Part model, mm, in its own coordinate system. A direction names the side the tool comes from. Coordinates: 2 decimals unless noted, no trailing zeros. Loops run counter-clockwise (first coordinate to the right, second up) from the corner with the lowest first, then second, coordinate; pieces in that order, holes last. Notation, with made-up numbers: M 72.5,19.25 L 128.5,19.25 A33 cw 128.5,57.25 Z; hole C 63.5,-14 d3. An arc over 180 degrees is marked long. Answer as a JSON object with one key per item and string values. Group by question number.
1. Drop flat-ended pins along their axis: pin 1 Ø0.6 at (y, z) = (4, -2.5) entering from -X; pin 2 Ø2 at (x, z) = (3, -2) entering from -Y; pin 3 Ø1.6 at (x, y) = (17, 5.5) entering from -Z. Give the stop position or say it passes through.
2. Mould opens along Y. For faces 6 (the face through (16.6, 2.7, -2.2)), 7 (the face through (17, 7, -2.2)) say: released by +Y, released by -Y, zero draft, split by the parting line, or undercut.
3. 3-axis set-ups, long thin cutter, end or side, ignore diameter. For faces 1 (the face through (1.6, 0.3, 3.05)), 2 (the face through (16.5, 5.3, -2.2)), 3 (the face through (16.5, 5.3, 2.2)), 4 (the face through (17, 7, 2.2)), 5 (the face through (1, 0, 2.75)): which of +Z, -Z, +X, -X, +Y, -Y reach the whole face in a straight line?
4. Drill centre lines: L1, parallel to Z at x = 17.5, y = 2.5; L2, parallel to Y at x = 16.55, z = 2.4; L3, parallel to Y at x = 1.65, z = 2.95. Where is each one in solid material? Low to high.
5. Saw through at D-D on x = 13.75. Write the cut outline in (y, z), then the cut area to 3 significant figures.
6. Saw through at C-C on y = 5.25. Write the cut outline in (x, z), then the cut area to 3 significant figures.
7. Saw through at B-B on y = -0.75. Write the cut outline in (x, z).
8. Saw through at A-A on z = 0.75. Write the cut outline in (x, y).
Autodesk Inventor part; units mm, degrees
ref_plane "YZ Plane" through (0, 0, 0) normal (1, 0, 0) x (0, 1, 0)
ref_plane "XZ Plane" through (0, 0, 0) normal (0, 1, 0) x (-1, 0, 0)
ref_plane "XY Plane" through (0, 0, 0) normal (0, 0, 1) x (1, 0, 0)
sketch "Sketch1" plane through (0, 0, 0) normal (1, 0, 0) x (0, 1, 0)
  line L0 (1.75, 3.05) -> (-2.05, 3.05)
  line L1 (-2.05, 3.05) -> (-2.05, 2.75)
  line L2 (-2.05, 2.75) -> (1.45, 2.75)
  line L3 (1.45, 2.75) -> (1.45, -2.75)
  line L4 (1.45, -2.75) -> (-2.05, -2.75)
  line L5 (-2.05, -2.75) -> (-2.05, -3.05)
  line L6 (-2.05, -3.05) -> (1.75, -3.05)
  line L7 (1.75, -3.05) -> (1.75, 3.05)
  point P0 (0, 0)
  dimension "d0" = 0.3
  dimension "d1" = 0.3
  dimension "d2" = 0.3
  dimension "d4" = 3.5
  dimension "d15" = 6.1
  dimension "d16" = 3.05
  dimension "d17" = 1.75
extrude "Extrusion1" add sketch "Sketch1" along normal blind 3.3
fillet "Fillet1" radius 1.6 4 edges at (3.3, -2.05, 2.9) (0, -2.05, 2.9) (0, -2.05, -2.9) (3.3, -2.05, -2.9)
sketch "Sketch2" plane through (0, 1.75, 3.05) normal (0, 0, 1) x (1, 0, 0)
  arc A0 (1.7, -3.8) -> (3.3, -2.2) centre (1.7, -2.2) ccw
  arc A1 (0, -2.2) -> (1.6, -3.8) centre (1.6, -2.2) ccw
  line L0 (1.6, -2.2) -> (1.7, -2.2)
  point P0 (0, -1.75)
  point P1 (1.65, -2.2)
hole "Hole1" at (1.65, -0.45, 3.05) direction (0, 0, -1) diameter 1 end through all
sketch "Sketch3" plane through (3.3, 0, 0) normal (1, 0, 0) x (0, 0, -1)
  line L0 (3.05, 1.75) -> (-3.05, 1.75)
  line L1 (0, 1.75) -> (0, 1.45)
  line L2 (-2.75, 1.45) -> (2.75, 1.45)
  line L3 (2, 1.45) -> (-2, 1.45)
  line L4 (-2, 1.45) -> (-2, 1.75)
  line L5 (-2, 1.75) -> (2, 1.75)
  line L6 (2, 1.75) -> (2, 1.45)
  line L7 (2, 1.45) -> (-2, 1.75) construction
  line L8 (-2, 1.45) -> (2, 1.75) construction
  point P0 (0, 0)
  point P1 (0, 1.6)
  dimension "d18" = 4
extrude "Extrusion2" add sketch "Sketch3" along normal blind 15.25
sketch "Sketch4" plane through (18.55, 0, 0) normal (1, 0, 0) x (0, 0, -1)
  line L0 (-2.75, 1.45) -> (2.75, 1.45)
  line L1 (0, 1.45) -> (0, 1.75)
  line L2 (3.05, 1.75) -> (-3.05, 1.75)
  line L3 (2.5, 1.45) -> (-2.5, 1.45)
  line L4 (-2.5, 1.45) -> (-2.5, 1.75)
  line L5 (-2.5, 1.75) -> (2.5, 1.75)
  line L6 (2.5, 1.75) -> (2.5, 1.45)
  line L7 (2.5, 1.45) -> (-2.5, 1.75) construction
  line L8 (-2.5, 1.45) -> (2.5, 1.75) construction
  line L9 (-2.5, 1.75) -> (-2.2, 1.75)
  line L10 (-2.2, 1.75) -> (-2.2, 6.75)
  line L11 (-2.2, 6.75) -> (-2.5, 6.75)
  line L12 (-2.5, 6.75) -> (-2.5, 1.75)
  line L13 (2.5, 1.75) -> (2.2, 1.75)
  line L14 (2.2, 1.75) -> (2.2, 6.75)
  line L15 (2.2, 6.75) -> (2.5, 6.75)
  line L16 (2.5, 6.75) -> (2.5, 1.75)
  point P0 (0, 0)
  point P1 (0, 1.6)
  dimension "d21" = 5
  dimension "d22" = 0.3
  dimension "d23" = 0.3
  dimension "d24" = 5
extrude "Extrusion3" add sketch "Sketch4" against normal blind 4
fillet "Fillet2" radius 2 4 edges at (18.55, 6.75, 2.35) (14.55, 6.75, 2.35) (14.55, 6.75, -2.35) (18.55, 6.75, -2.35)
sketch "Sketch5" plane through (14.55, 1.45, 2.5) normal (0, 0, 1) x (1, 0, 0)
  arc A0 (4, 3.3) -> (0, 3.3) centre (2, 3.3) ccw
  point P0 (-14.55, -1.45)
  point P1 (2, 3.8)
  dimension "d35" = 0.5
hole "Hole2" at (16.55, 5.25, 2.5) direction (0, 0, -1) diameter 1 end through all
sketch "Sketch6" plane through (14.55, 1.75, -2.2) normal (0, 0, 1) x (1, 0, 0)
  circle A0 centre (2, 3.5) radius 0.5
  circle A1 centre (2, 3.5) radius 0.5
  circle A2 centre (2, 3.5) radius 2.25
  point P0 (-14.55, -1.75)
  dimension "d36" = 4.5
extrude "Extrusion4" add sketch "Sketch6" along normal blind 4.4 contours A0 | A2
ref_plane "Work Plane1" through (-1.2438, 1.2458, -3.05) normal (-0.9978, 0.0664, 0) x (-0.0664, -0.9978, 0)
sketch "Sketch7" plane through (-1.2438, 1.2458, -3.05) normal (-0.9978, 0.0664, 0) x (-0.0664, -0.9978, 0)
  circle A0 centre (-6.8395, 3.05) radius 0.875
  point P0 (1.1605, 3.05)
  dimension "d39" = 1.75
  dimension "d40" = 8
properties part number "Arm"
Outcome:
{
 "1": {"pin 1": "stops at x = 14.55", "pin 2": "stops at y = -1.92", "pin 3": "stops at z = -2.5"},
 "2": {"face 6": "undercut", "face 7": "zero draft"},
 "3": {"face 1": "+Z, +X, -X, +Y, -Y", "face 2": "-Z", "face 3": "+Z", "face 4": "+Z, +Y", "face 5": "+X, -X, -Y"},
 "4": {"L1": "z = -2.5 to -2.2, 2.2 to 2.5", "L2": "y = 1.45 to 4.75, 5.75 to 6.75", "L3": "y = -2.05 to -0.95, 0.05 to 1.75"},
 "5": {"outline": "M 1.45,-2 L 1.75,-2 L 1.75,2 L 1.45,2 Z", "area": "1.20 mm²"},
 "6": {"outline": "M 14.3,-2.2 L 14.61,-2.2 L 14.61,-2.5 L 16.05,-2.5 L 16.05,-2.2 L 17.05,-2.2 L 17.05,-2.5 L 18.49,-2.5 L 18.49,-2.2 L 18.8,-2.2 L 18.8,2.2 L 18.49,2.2 L 18.49,2.5 L 17.05,2.5 L 17.05,2.2 L 16.05,2.2 L 16.05,2.5 L 14.61,2.5 L 14.61,2.2 L 14.3,2.2 Z", "area": "21.5 mm²"},
 "7": {"outline": "M 0.03,-3.05 L 1.25,-3.05 L 1.25,-2.75 L 0.03,-2.75 Z; M 0.03,2.75 L 1.25,2.75 L 1.25,3.05 L 0.03,3.05 Z; M 2.05,-3.05 L 3.27,-3.05 L 3.27,-2.75 L 2.05,-2.75 Z; M 2.05,2.75 L 3.27,2.75 L 3.27,3.05 L 2.05,3.05 Z"},
 "8": {"outline": "M 0,1.45 L 18.55,1.45 L 18.55,1.75 L 0,1.75 Z; C 16.55,5.25 d4.5"}
}
